from build123d import *

# Parameters (mm, degrees)
SKIZZE1_W                       = 7
SKIZZE1_H                       = 7
AUFSATZ_LINEAR_AUSTRAGEN1_DEPTH = 15
SKIZZE2_W                       = 3.1
SKIZZE2_H                       = 3.4
SCHNITT_LINEAR_AUSTRAGEN1_DEPTH = 16.795568999
SKIZZE3_W                       = 5
SKIZZE3_H                       = 10
SCHNITT_LINEAR_AUSTRAGEN2_DEPTH = 5
FASE2_SIZE                      = 1
FASE2_SIZE2                     = 1.732050808
SKIZZE5_W                       = 3.5
SKIZZE5_H                       = 10
AUFSATZ_LINEAR_AUSTRAGEN2_DEPTH = 10
FASE3_SIZE                      = 1
SKIZZE6_R                       = 2.65
SCHNITT_LINEAR_AUSTRAGEN3_DEPTH = 10
FASE4_SIZE                      = 1


with BuildPart() as part:
    # Skizze1 → Aufsatz-Linear austragen1 (new body)
    with BuildSketch(Plane.XY):
        Rectangle(SKIZZE1_W, SKIZZE1_H)
    extrude(amount=AUFSATZ_LINEAR_AUSTRAGEN1_DEPTH)

    # Skizze2 → Schnitt-Linear austragen1 (cut, through all)
    with BuildSketch(Plane.XY.offset(15)):
        Rectangle(SKIZZE2_W, SKIZZE2_H)
    extrude(amount=-SCHNITT_LINEAR_AUSTRAGEN1_DEPTH, mode=Mode.SUBTRACT)

    # Skizze3 → Schnitt-Linear austragen2 (cut)
    with BuildSketch(Plane(origin=(0, 3.5, 0), x_dir=(1, 0, 0), z_dir=(0, 1, 0))):
        with Locations((1, -7.5)):
            Rectangle(SKIZZE3_W, SKIZZE3_H)
    extrude(amount=-SCHNITT_LINEAR_AUSTRAGEN2_DEPTH, mode=Mode.SUBTRACT)

    # Fase2
    fase2_edges = [part.edges().sort_by_distance(p)[0] for p in [
        (-1.5, 3.5, 7.5),
    ]]
    fase2_side = [part.faces().sort_by_distance(p)[0] for p in [
        (0, 3.5, 0.165529454),
    ]]
    chamfer(fase2_edges, length=FASE2_SIZE, length2=FASE2_SIZE2, reference=fase2_side[0])

    # Skizze5 → Aufsatz-Linear austragen2 (add)
    with BuildSketch(Plane.XZ.offset(3.5)):
        with Locations((-1.75, 7.5)):
            Rectangle(SKIZZE5_W, SKIZZE5_H)
    extrude(amount=AUFSATZ_LINEAR_AUSTRAGEN2_DEPTH)

    # Fase3
    fase3_edges = [part.edges().sort_by_distance(p)[0] for p in [
        (-1.75, -3.5, 2.5),
        (0, -3.5, 7.5),
        (-1.75, -3.5, 12.5),
    ]]
    chamfer(fase3_edges, length=FASE3_SIZE)

    # Skizze6 → Schnitt-Linear austragen3 (cut)
    with BuildSketch(Plane(origin=(0, 0, 0), x_dir=(0, 0, -1), z_dir=(1, 0, 0))):
        with Locations((-7.5, -9)):
            Circle(SKIZZE6_R)
    extrude(amount=-SCHNITT_LINEAR_AUSTRAGEN3_DEPTH, mode=Mode.SUBTRACT)

    # Fase4
    fase4_edges = [part.edges().sort_by_distance(p)[0] for p in [
        (3.5, -1.5, 7.5),
    ]]
    chamfer(fase4_edges, length=FASE4_SIZE)


solid = part.part
Input: part model. Units: mm. Frame: model coordinates. A direction names the side the tool comes from. Coordinates: 2 decimals unless noted, no trailing zeros. Loops run counter-clockwise (first coordinate to the right, second up) from the corner with the lowest first, then second, coordinate; pieces in that order, holes last.
Q1. Set-up query: faces 1 (the face through (0, 1.7, 13)), 2 (the face through (0, -11, 10)), 3 (the face through (-1.99, 2.62, 7.57)), 4 (the face through (2, -3.5, 7)). Return all of +Z, -Z, +X, -X, +Y, -Y with unobstructed straight access to the full face (end or side cutting, diameter ignored); none if empty.
Q2. Contact query for flat-ended pins moving along their axis: pin 1 (3 mm diameter, centred on x = -2.5, y = -11, fed in from +Z); pin 2 (0.5 mm diameter, centred on x = 2, z = 6.5, fed in from +Y); pin 3 (4 mm diameter, centred on x = -2, y = -9, fed in from -Z). Output: stop coordinate, or through.
Q3. Cut plane A-A (y = 1). Output: boundary loops of the cut face in (x, z), then the cut area to 3 significant figures.
Q4. Cut plane C-C (y = -9). Output: boundary loops of the cut face in (x, z).
Q5. Cut plane B-B (z = 7.5). Output: boundary loops of the cut face in (x, y), then the cut area to 3 significant figures.
Q6. Cut plane D-D (x = -3). Output: boundary loops of the cut face in (y, z).
Q7. Material intervals for line 1 (Y direction, x = 0, z = 1.25); line 2 (Y direction, x = -1.05, z = 7.5); line 3 (X direction, y = -5.25, z = 11.5), sorted ascending.
Q8. Draft query along Y for faces 5 (the face through (-2, -9, 12.5)), 6 (the face through (1.55, 0, 13)), 7 (the face through (0.5, -4, 7.4)). Return one class per face: +Y half, -Y half, draft (parallel to the pull), parting line (faces both ways), or undercut.
Working result:
1. face 1: +Z, -Z
1. face 2: +Z, -Z, +X, -Y
1. face 3: +X, +Y
1. face 4: +X, -Y
2. pin 1: stops at z = 12.5
2. pin 2: stops at y = -1.5
2. pin 3: stops at z = 2.5
3. outline: (-3.5, 0) - (-1.55, 0) - (-1.55, 15) - (-3.5, 15) - close; (1.55, 0) - (3.5, 0) - (3.5, 2.5) - (1.55, 2.5) - close; (1.55, 12.5) - (3.5, 12.5) - (3.5, 15) - (1.55, 15) - close
3. area: 39.0 mm2
4. outline: (-3.5, 2.5) - (0, 2.5) - (0, 4.85) - (-3.5, 4.85) - close; (-3.5, 10.15) - (0, 10.15) - (0, 12.5) - (-3.5, 12.5) - close
5. outline: (-3.5, -13.5) - (0, -13.5) - (0, -11.65) - (-3.5, -11.65) - close; (-3.5, -6.35) - (0, -6.35) - (0, -4.5) - (1, -3.5) - (3.5, -3.5) - (3.5, -2.5) - (2.5, -1.5) - (1.55, -1.5) - (1.55, -1.7) - (-1.55, -1.7) - (-1.55, 1.7) - (-1.5, 1.7) - (-1.5, 1.77) - (-2.5, 3.5) - (-3.5, 3.5) - close
5. area: 38.8 mm2
6. outline: (-13.5, 2.5) - (-4.5, 2.5) - (-3.5, 1.5) - (-3.5, 0) - (3.5, 0) - (3.5, 15) - (-3.5, 15) - (-3.5, 13.5) - (-4.5, 12.5) - (-13.5, 12.5) - close; hole circle Ø5.3 at (-9, 7.5)
7. line 1: y = -3.5 to -1.7, 1.7 to 3.5
7. line 2: y = -13.5 to -11.65, -6.35 to -1.7
7. line 3: x = -3.5 to 0
8. face 5: draft
8. face 6: undercut
8. face 7: -Y half
